```python
from build123d import *

# Parameters (mm, degrees)
F1_R     = 38.1
F1_R_2   = 26.9875
F1_R_3   = 20.6375
F2_DEPTH = 38.1
F3_DEPTH = 30.1625
F4_R     = 8.7249
F5_DEPTH = 254
F6_R     = 2.3749
F7_DEPTH = 50.8


with BuildPart() as f2:
    # F1 (on Top) → F2 (new body, symmetric)
    with BuildSketch(Plane.XY):
        Circle(F1_R)
        Circle(F1_R_2, mode=Mode.SUBTRACT)
        Circle(F1_R_2)
        Circle(F1_R_3, mode=Mode.SUBTRACT)
    extrude(amount=F2_DEPTH, both=True)

    # F0 (on Top) → F3 (join, symmetric)
    with BuildSketch(Plane.XY):
        with BuildLine():
            ThreePointArc((38.1, 0), (26.940768, -26.940768), (0, -38.1))
            Line((0, -38.1), (0, -73.025))
            Line((0, -73.025), (41.052193, -73.025))
            ThreePointArc((41.052193, -73.025), (43.297257, -73.954936), (44.227193, -76.2))
            Line((44.227193, -76.2), (88.677193, -76.2))
            Line((88.677193, -76.2), (88.677193, -60.325))
            ThreePointArc((88.677193, -60.325), (86.817321, -55.834872), (82.327193, -53.975))
            Line((82.327193, -53.975), (47.625, -53.975))
            ThreePointArc((47.625, -53.975), (40.889808, -51.185192), (38.1, -44.45))
            Line((38.1, -44.45), (38.1, 0))
        make_face()
        with BuildLine():
            Line((0, -73.025), (0, -38.1))
            ThreePointArc((0, -38.1), (-26.940768, -26.940768), (-38.1, 0))
            Line((-38.1, 0), (-38.1, -44.45))
            ThreePointArc((-38.1, -44.45), (-40.889808, -51.185192), (-47.625, -53.975))
            Line((-47.625, -53.975), (-82.772807, -53.975))
            ThreePointArc((-82.772807, -53.975), (-87.262935, -55.834872), (-89.122807, -60.325))
            Line((-89.122807, -60.325), (-89.122807, -76.2))
            Line((-89.122807, -76.2), (-44.672807, -76.2))
            ThreePointArc((-44.672807, -76.2), (-43.742871, -73.954936), (-41.497807, -73.025))
            Line((-41.497807, -73.025), (0, -73.025))
        make_face()
    extrude(amount=F3_DEPTH, both=True)

    # F4 (on Front) → F5 (cut)
    with BuildSketch(Plane.XZ):
        with Locations((-66.675, 0)):
            Circle(F4_R)
        with Locations((66.675, 0)):
            Circle(F4_R)
    extrude(amount=F5_DEPTH, mode=Mode.SUBTRACT)

    # F6 (on Front) → F7 (cut)
    with BuildSketch(Plane.XZ):
        Circle(F6_R)
    extrude(amount=-F7_DEPTH, mode=Mode.SUBTRACT)


solid = f2.part
```
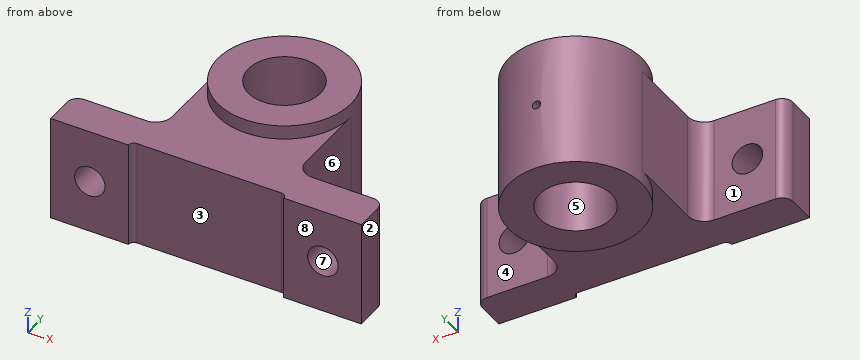
The model under review builds one solid part; all positions refer to its coordinate system, in mm. Face numbers are marked on the shaded views. A direction names the side the tool comes from. Round coordinates to 2 decimals unless told otherwise and drop trailing zeros. Loops run counter-clockwise (first coordinate to the right, second up) from the corner with the lowest first, then second, coordinate; pieces in that order, holes last. Notation, with made-up numbers: (-25.75, 57.5) - (-1.75, 57.5) arc R28 ccw to (-1.75, 83.5) - close; hole circle Ø2 at (70, 25.5). An arc over 180 degrees is marked (long way). Use a Markdown table: item, result. Add a question column.
Q1. Add section D-D (z = 0). State how many separate pieces and enclosed holes the cut face has, plus the area to 3 significant figures.
Q2. For probe 1 along X at (y, z) = (-68, 0); probe 2 along Y at (x, z) = (0, -20.5) (1 decimal); probe 3 along X at (y, z) = (32, 0), list the stretches that pass through material, from the lowest coordinate up.
Q3. Add section B-B (x = 0). State the section outline as (y, z) points (1 decimal).
Q4. The part is to be moulded in two halves that separate along X. For the marked faces 5, 6, 7 and 8, say which applies: pulls with the +X half, pulls with the -X half, needs draft (parallel to the pull), parting line crosses it, or undercut.
Q5. Add section C-C (y = -6.5). State the section outline as (x, z) points.
Q6. Insertion check: pin 1 Ø22.5 at (x, z) = (-66.675, 0) entering from -Y; pin 2 Ø5.5 at (x, z) = (0, 0) entering from -Y (3 decimals); pin 3 Ø12 at (x, y) = (-5.5, -55.5) entering from -Z; pin 4 Ø1.5 at (y, z) = (-34, 14.5) entering from +X. Each pin has a flat end and moves straight along its axis. Give the tip position at first contact, or say it passes through.
Q7. Machinability: for the marked faces 1, 2, 3 and 4, which of the approach directions +Z, -Z, +X, -X, +Y, -Y give a long, thin tool a straight path to every point of the face, cutting with its end or side? Answer none if there is none.
Worked answers:
| question | item | result |
|---|---|---|
| 1 | separate pieces | 3 |
| 1 | enclosed holes | 0 |
| 1 | area | 7,890 mm² |
| 2 | probe 1 | -89.12 to -75.4, -57.95 to 57.95, 75.4 to 88.68 |
| 2 | probe 2 | -73 to -20.6, 20.6 to 38.1 |
| 2 | probe 3 | -20.68 to -2.37, 2.37 to 20.68 |
| 3 | outline | (-73, -30.2) - (-38.1, -30.2) - (-38.1, -38.1) - (-20.6, -38.1) - (-20.6, 38.1) - (-38.1, 38.1) - (-38.1, 30.2) - (-73, 30.2) - close; (20.6, -38.1) - (38.1, -38.1) - (38.1, -2.4) - (20.6, -2.4) - close; (20.6, 2.4) - (38.1, 2.4) - (38.1, 38.1) - (20.6, 38.1) - close |
| 4 | face 5 | undercut |
| 4 | face 6 | pulls with the +X half |
| 4 | face 7 | undercut |
| 4 | face 8 | needs draft |
| 5 | outline | (-38.1, -30.16) - (-37.54, -30.16) - (-37.54, -38.1) - (-19.59, -38.1) - (-19.59, 38.1) - (-37.54, 38.1) - (-37.54, 30.16) - (-38.1, 30.16) - close; (19.59, -38.1) - (37.54, -38.1) - (37.54, -30.16) - (38.1, -30.16) - (38.1, 30.16) - (37.54, 30.16) - (37.54, 38.1) - (19.59, 38.1) - close |
| 6 | pin 1 | y = -76.2 |
| 6 | pin 2 | y = -73.025 |
| 6 | pin 3 | z = -30.16 |
| 6 | pin 4 | x = 38.1 |
| 7 | face 1 | +Z, -Z, -X, +Y |
| 7 | face 2 | +Z, -Z, +X, +Y, -Y |
| 7 | face 3 | +Z, -Z, -Y |
| 7 | face 4 | +Z, -Z, +X, +Y |
